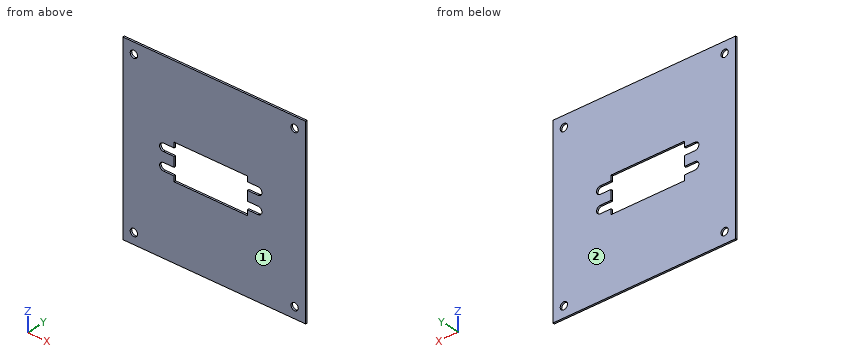
from build123d import *

# Parameters (mm, degrees)
SKETCH1_W          = 102.4
SKETCH1_H          = 102.4
SKETCH1_R          = 2.05
SKETCH1_W_2        = 41
SKETCH1_H_2        = 20
BASE_FLANGE1_DEPTH = 1
CUT_EXTRUDE2_DEPTH = 10


# Sheet-metal steps are written as plain solids
with BuildPart() as part:
    # Sketch1 → Base-Flange1 (new body)
    with BuildSketch(Plane(origin=(0, 0, 0), x_dir=(1, 0, 0), z_dir=(0, 1, 0))):
        Rectangle(SKETCH1_W, SKETCH1_H)
        with Locations(Location((45.02, 45.02, 0), (0, 0, 270))):
            Circle(SKETCH1_R, mode=Mode.SUBTRACT)
        with Locations(Location((45.02, -45.02, 0), (0, 0, 270))):
            Circle(SKETCH1_R, mode=Mode.SUBTRACT)
        with Locations(Location((-45.02, -45.02, 0), (0, 0, 270))):
            Circle(SKETCH1_R, mode=Mode.SUBTRACT)
        with Locations(Location((-45.02, 45.02, 0), (0, 0, 270))):
            Circle(SKETCH1_R, mode=Mode.SUBTRACT)
        with Locations((-1.95, 0)):
            Rectangle(SKETCH1_W_2, SKETCH1_H_2, mode=Mode.SUBTRACT)
    extrude(amount=-BASE_FLANGE1_DEPTH)

    # Sketch7 → Cut-Extrude2 (cut)
    with BuildSketch(Plane(origin=(0, 0, 0), x_dir=(1, 0, 0), z_dir=(0, 1, 0))):
        with BuildLine():
            Line((-28.45, 7.05), (-16.45, 7.05))
            ThreePointArc((-16.45, 7.05), (-14.3, 4.9), (-16.45, 2.75))
            Line((-16.45, 2.75), (-28.45, 2.75))
            ThreePointArc((-28.45, 2.75), (-30.6, 4.9), (-28.45, 7.05))
        make_face()
        with BuildLine():
            Line((-28.45, -2.75), (-16.45, -2.75))
            ThreePointArc((-16.45, -2.75), (-14.3, -4.9), (-16.45, -7.05))
            Line((-16.45, -7.05), (-28.45, -7.05))
            ThreePointArc((-28.45, -7.05), (-30.6, -4.9), (-28.45, -2.75))
        make_face()
        with BuildLine():
            Line((12.55, 7.05), (24.55, 7.05))
            ThreePointArc((24.55, 7.05), (26.7, 4.9), (24.55, 2.75))
            Line((24.55, 2.75), (12.55, 2.75))
            ThreePointArc((12.55, 2.75), (10.4, 4.9), (12.55, 7.05))
        make_face()
        with BuildLine():
            Line((12.55, -2.75), (24.55, -2.75))
            ThreePointArc((24.55, -2.75), (26.7, -4.9), (24.55, -7.05))
            Line((24.55, -7.05), (12.55, -7.05))
            ThreePointArc((12.55, -7.05), (10.4, -4.9), (12.55, -2.75))
        make_face()
    extrude(amount=-CUT_EXTRUDE2_DEPTH, mode=Mode.SUBTRACT)


solid = part.part
Can you work these out from the model? Positions are in its coordinate system, mm. Face numbers are marked on the shaded views. Coordinates: 2 decimals unless noted, no trailing zeros. Write each loop counter-clockwise with the first axis right and the second up, starting at its lowest first coordinate (ties: lowest second). Pieces come first, ordered by that corner, then holes. Notation, with made-up numbers: M 15,-27.75 L 26,-27.75 A18 ccw 26,2.25 Z; hole C 36,1.5 d2. An arc over 180 degrees is marked long. Use one line per item in the form item = value.
Q1. If we section it at B-B (x = 20): Write out the boundary of the cut face in (y, z), then the cut area to 3 significant figures.
Model answer:
outline = M -1,-51.2 L 0,-51.2 L 0,-7.05 L -1,-7.05 Z; M -1,-2.75 L 0,-2.75 L 0,2.75 L -1,2.75 Z; M -1,7.05 L 0,7.05 L 0,51.2 L -1,51.2 Z
area = 93.8 mm^2
Q2. I need wall thicknesses on line 1 along Z through (x, y) = (21.5, -0.8); line 2 along X through (y, z) = (-0.7, -45.02); line 3 along X through (y, z) = (-0.2, 44). Which ranges of each line are inside material? Lowest first, please. Write a range as from..to.
Model answer:
line_1 = -51.2..-7.05, -2.75..2.75, 7.05..51.2
line_2 = -51.2..-47.07, -42.97..42.97, 47.07..51.2
line_3 = -51.2..-46.8, -43.24..43.24, 46.8..51.2
Q3. If we section it at D-D (z = 4.9): Write out the boundary of the cut face in (x, y).
Model answer:
outline = M -51.2,-1 L -30.6,-1 L -30.6,0 L -51.2,0 Z; M 26.7,-1 L 51.2,-1 L 51.2,0 L 26.7,0 Z
Q4. If we section it at A-A (z = -45.02): Write out the boundary of the cut face in (x, y), then the cut area to 3 significant figures.
Model answer:
outline = M -51.2,-1 L -47.07,-1 L -47.07,0 L -51.2,0 Z; M -42.97,-1 L 42.97,-1 L 42.97,0 L -42.97,0 Z; M 47.07,-1 L 51.2,-1 L 51.2,0 L 47.07,0 Z
area = 94.2 mm^2
Q5. We'd pull the mould along Y, two halves only. Please class the marked faces 1 and 2: +Y half, -Y half, draft (parallel to the pull), parting line (faces both ways), or undercut.
Model answer:
face_1 = -Y half
face_2 = +Y half
Q6. If we section it at C-C (y = -0.35): Write out the boundary of the cut face in (x, z), then the cut area to 3 significant figures.
Model answer:
outline = M -51.2,-51.2 L 51.2,-51.2 L 51.2,51.2 L -51.2,51.2 Z; hole C -45.02,-45.02 d4.1; hole C -45.02,45.02 d4.1; hole M -28.45,-7.05 L -22.45,-7.05 L -22.45,-10 L 18.55,-10 L 18.55,-7.05 L 24.55,-7.05 A2.15 ccw 24.55,-2.75 L 18.55,-2.75 L 18.55,2.75 L 24.55,2.75 A2.15 ccw 24.55,7.05 L 18.55,7.05 L 18.55,10 L -22.45,10 L -22.45,7.05 L -28.45,7.05 A2.15 ccw -28.45,2.75 L -22.45,2.75 L -22.45,-2.75 L -28.45,-2.75 A2.15 ccw Z; hole C 45.02,-45.02 d4.1; hole C 45.02,45.02 d4.1
area = 9,480 mm^2
Q7. For P1, Ø2, axis at x = 27, z = -36.5, coming from the +Y side; P2, Ø2.5, axis at x = -45.02, z = 45.02, coming from the -Y side, each with a flat end and sliding along its axis, tell me the tip position at first contact or that it passes through.
Model answer:
P1 = 0
P2 = through
